from build123d import *

# Parameters (mm, degrees)
BOSS_EXTRUDE1_DEPTH        = 4
BOSS_EXTRUDE1_DEPTH_BACK   = 4
SKETCH1_R                  = 3.5
BOSS_EXTRUDE1_2_DEPTH      = 4
BOSS_EXTRUDE1_2_DEPTH_BACK = 4
SKETCH1_R_2                = 22
SKETCH1_R_3                = 19
BOSS_EXTRUDE2_DEPTH        = 1.5
BOSS_EXTRUDE2_DEPTH_BACK   = 1.5
SKETCH1_3_R                = 19
SKETCH1_3_R_2              = 3.5


with BuildPart() as part:
    # Sketch1 → Boss-Extrude1 (new, two sides: drawn at the far end of the back side and taken through both)
    with BuildSketch(Plane.XY.offset(-BOSS_EXTRUDE1_DEPTH_BACK)):
        Circle(SKETCH1_R)
        with BuildLine():
            ThreePointArc((1.118033989, -1), (0, 1.5), (-1.118033989, -1))
            Line((-1.118033989, -1), (1.118033989, -1))
        make_face(mode=Mode.SUBTRACT)
    extrude(amount=BOSS_EXTRUDE1_DEPTH + BOSS_EXTRUDE1_DEPTH_BACK)



with BuildPart() as body_2:
    # Sketch1 → Boss-Extrude1 2 (new, two sides: drawn at the far end of the back side and taken through both)
    with BuildSketch(Plane.XY.offset(-BOSS_EXTRUDE1_2_DEPTH_BACK)):
        Circle(SKETCH1_R_2)
        Circle(SKETCH1_R_3, mode=Mode.SUBTRACT)
    extrude(amount=BOSS_EXTRUDE1_2_DEPTH + BOSS_EXTRUDE1_2_DEPTH_BACK)


with BuildPart() as part_1:
    add(part.part)

    add(body_2.part)  # Boss-Extrude2 merges body 2
    # Sketch1_3 → Boss-Extrude2 (add, two sides: drawn at the far end of the back side and taken through both)
    with BuildSketch(Plane.XY.offset(-BOSS_EXTRUDE2_DEPTH_BACK)):
        Circle(SKETCH1_3_R)
        Circle(SKETCH1_3_R_2, mode=Mode.SUBTRACT)
    extrude(amount=BOSS_EXTRUDE2_DEPTH + BOSS_EXTRUDE2_DEPTH_BACK)


solid = part_1.part
Could you check a few things on this model? Use its own coordinates, in mm. A direction names the side the tool comes from. Coordinates: 2 decimals unless noted, no trailing zeros. Loops run counter-clockwise (first coordinate to the right, second up) from the corner with the lowest first, then second, coordinate; pieces in that order, holes last. Notation, with made-up numbers: (-30.75, 23.25) -> (-2.75, 23.25) arc R35 ccw to (-2.75, 57.25) -> close; hole circle Ø4 at (9, 60.5). An arc over 180 degrees is marked (long way). Answer in a Markdown table with one row per item.
(1) Imagine slicing it at A-A (z = -2.5). List the corners of the cut face in (x, y) for me.
Results found:
| item | result |
|---|---|
| outline | circle Ø44 at (0, 0); circle Ø7 at (0, 0); hole circle Ø38 at (0, 0); hole (-1.12, -1) -> (1.12, -1) arc R1.5 ccw (long way) to start |
(2) Imagine slicing it at C-C (x = 0). List the corners of the cut face in (y, z) for me, plus the area to 3 significant figures.
Results found:
| item | result |
|---|---|
| outline | (-22, -4) -> (-19, -4) -> (-19, -1.5) -> (-3.5, -1.5) -> (-3.5, -4) -> (-1, -4) -> (-1, 4) -> (-3.5, 4) -> (-3.5, 1.5) -> (-19, 1.5) -> (-19, 4) -> (-22, 4) -> close; (1.5, -4) -> (3.5, -4) -> (3.5, -1.5) -> (19, -1.5) -> (19, -4) -> (22, -4) -> (22, 4) -> (19, 4) -> (19, 1.5) -> (3.5, 1.5) -> (3.5, 4) -> (1.5, 4) -> close |
| area | 177 mm^2 |
(3) Thinking about a two-plate mould opening in Y: for faces 5 (the face through (-4.769, -21.477, -0.056)), 6 (the face through (0, -4, 1.5)), 7 (the face through (0, -2, -4)), which applies, released by +Y, released by -Y, zero draft, split by the parting line, or undercut?
Results found:
| item | result |
|---|---|
| face 5 | split by the parting line |
| face 6 | undercut |
| face 7 | zero draft |
(4) If I drill on probe 1 along Y at (x, z) = (-2.5, -3); probe 2 along Y at (x, z) = (-0.5, 3); probe 3 along X at (y, z) = (15, 3), over which ranges is the centre line in solid material (lowest first)?
Results found:
| item | result |
|---|---|
| probe 1 | y = -21.86 to -18.83, -2.45 to 2.45, 18.83 to 21.86 |
| probe 2 | y = -21.99 to -18.99, -3.46 to -1, 1.41 to 3.46, 18.99 to 21.99 |
| probe 3 | x = -16.09 to -11.66, 11.66 to 16.09 |
(5) Imagine slicing it at D-D (y = 6.5). List the corners of the cut face in (x, z) for me.
Results found:
| item | result |
|---|---|
| outline | (-21.02, -4) -> (-17.85, -4) -> (-17.85, -1.5) -> (17.85, -1.5) -> (17.85, -4) -> (21.02, -4) -> (21.02, 4) -> (17.85, 4) -> (17.85, 1.5) -> (-17.85, 1.5) -> (-17.85, 4) -> (-21.02, 4) -> close |
(6) Will these pins go through, and if not, where does the flat tip stop? pin 1 Ø1 at (y, z) = (-4, 1.5) entering from -X; pin 2 Ø1.5 at (y, z) = (-6, 3) entering from +X; pin 3 Ø2.5 at (x, z) = (0, 0.5) entering from +Y.
Results found:
| item | result |
|---|---|
| pin 1 | stops at x = -21.72 |
| pin 2 | stops at x = 21.36 |
| pin 3 | stops at y = 22 |
(7) For faces 1 (the face through (-7, 18, 4)), 2 (the face through (0, -1, 0)), 3 (the face through (0, -4, -1.5)), 4 (the face through (3.233, -1.341, 2.732)), which set-ups out of +Z, -Z, +X, -X, +Y, -Y let a thin tool reach every point of the face, with its end or its side?
Results found:
| item | result |
|---|---|
| face 1 | +Z, +X, -X, +Y, -Y |
| face 2 | +Z, -Z |
| face 3 | -Z |
| face 4 | +Z |
(8) Imagine slicing it at B-B (y = 0). List the corners of the cut face in (x, z) for me.
Results found:
| item | result |
|---|---|
| outline | (-22, -4) -> (-19, -4) -> (-19, -1.5) -> (-3.5, -1.5) -> (-3.5, -4) -> (-1.5, -4) -> (-1.5, 4) -> (-3.5, 4) -> (-3.5, 1.5) -> (-19, 1.5) -> (-19, 4) -> (-22, 4) -> close; (1.5, -4) -> (3.5, -4) -> (3.5, -1.5) -> (19, -1.5) -> (19, -4) -> (22, -4) -> (22, 4) -> (19, 4) -> (19, 1.5) -> (3.5, 1.5) -> (3.5, 4) -> (1.5, 4) -> close |
